For this review, take the finished solid that the model builds, in its own axes (mm). Round coordinates to 2 decimals unless told otherwise and drop trailing zeros. Order: outer loops, then holes, each group sorted by start corner. A loop starts at its lowest first (then second) coordinate and runs counter-clockwise, first axis right, second up.
```python
from build123d import *

# Parameters (mm, degrees)
SKETCH_1_R          = 1.5
EXTRUDE_1_DEPTH     = 1
SKETCH_3_R          = 1.5
CUT_EXTRUDE_1_DEPTH = 61.191781662
SKETCH_4_R          = 1.5
CUT_EXTRUDE_2_DEPTH = 61.191781662
CUT_EXTRUDE_3_DEPTH = 61.191781662


with BuildPart() as part:
    # Эскиз1 → Бобышка-Вытянуть1 (new body)
    with BuildSketch(Plane(origin=(0, 0, 0), x_dir=(1, 0, 0), z_dir=(0, 1, 0))):
        with BuildLine():
            Line((-48, -36.304966321), (48, -36.304966321))
            Line((48, -36.304966321), (48, 6.254720986))
            ThreePointArc((48, 6.254720986), (47.707106781, 6.961827767), (47, 7.254720986))
            Line((47, 7.254720986), (36.5, 7.254720986))
            ThreePointArc((36.5, 7.254720986), (29.428932188, 10.183653174), (26.5, 17.254720986))
            Line((26.5, 17.254720986), (26.5, 22.788381883))
            ThreePointArc((26.5, 22.788381883), (29.428932188, 29.859449695), (36.5, 32.788381883))
            Line((36.5, 32.788381883), (47, 32.788381883))
            ThreePointArc((47, 32.788381883), (47.707106781, 33.081275101), (48, 33.788381883))
            Line((48, 33.788381883), (48, 35.304966322))
            ThreePointArc((48, 35.304966322), (47.707106781, 36.012073103), (47, 36.304966322))
            Line((47, 36.304966322), (-47, 36.304966322))
            ThreePointArc((-47, 36.304966322), (-47.707106781, 36.012073103), (-48, 35.304966322))
            Line((-48, 35.304966322), (-48, 33.788381883))
            ThreePointArc((-48, 33.788381883), (-47.707106781, 33.081275101), (-47, 32.788381883))
            Line((-47, 32.788381883), (-36.5, 32.788381883))
            ThreePointArc((-36.5, 32.788381883), (-29.428932188, 29.859449695), (-26.5, 22.788381883))
            Line((-26.5, 22.788381883), (-26.5, 17.254720986))
            ThreePointArc((-26.5, 17.254720986), (-29.428932188, 10.183653174), (-36.5, 7.254720986))
            Line((-36.5, 7.254720986), (-47, 7.254720986))
            ThreePointArc((-47, 7.254720986), (-47.707106781, 6.961827767), (-48, 6.254720986))
            Line((-48, 6.254720986), (-48, -36.304966321))
        make_face()
        with Locations(Location((-21.397134942, 13.404966321, 0), (0, 0, 270))):
            Circle(SKETCH_1_R, mode=Mode.SUBTRACT)
        with Locations(Location((-21.397134942, 33.804966321, 0), (0, 0, 270))):
            Circle(SKETCH_1_R, mode=Mode.SUBTRACT)
        with Locations(Location((22.502865058, 13.404966321, 0), (0, 0, 270))):
            Circle(SKETCH_1_R, mode=Mode.SUBTRACT)
        with Locations(Location((22.502865058, 33.804966321, 0), (0, 0, 270))):
            Circle(SKETCH_1_R, mode=Mode.SUBTRACT)
        with BuildLine():
            Line((-19.5, -0.787211353), (-18, -1.787211353))
            Line((-18, -1.787211353), (18, -1.787211353))
            Line((18, -1.787211353), (19.5, -0.787211353))
            Line((19.5, -0.787211353), (19.5, 6.212788647))
            ThreePointArc((19.5, 6.212788647), (20.378679656, 8.334108991), (22.5, 9.212788647))
            Line((22.5, 9.212788647), (23.024503903, 9.212788647))
            ThreePointArc((23.024503903, 9.212788647), (24.348525199, 8.904807891), (25.400697774, 8.044100386))
            Line((25.400697774, 8.044100386), (32.206912135, -0.787211353))
            Line((32.206912135, -0.787211353), (37, -0.787211353))
            ThreePointArc((37, -0.787211353), (39.121320344, -1.665891009), (40, -3.787211353))
            Line((40, -3.787211353), (40, -8.287211353))
            Line((40, -8.287211353), (38, -10.787211353))
            Line((38, -10.787211353), (38, -20.787211353))
            Line((38, -20.787211353), (40, -23.287211353))
            Line((40, -23.287211353), (40, -27.787211353))
            ThreePointArc((40, -27.787211353), (39.121320344, -29.908531696), (37, -30.787211353))
            Line((37, -30.787211353), (19.5, -30.787211353))
            Line((19.5, -30.787211353), (18, -29.787211353))
            Line((18, -29.787211353), (-18, -29.787211353))
            Line((-18, -29.787211353), (-19.5, -30.787211353))
            Line((-19.5, -30.787211353), (-37, -30.787211353))
            ThreePointArc((-37, -30.787211353), (-39.121320344, -29.908531696), (-40, -27.787211353))
            Line((-40, -27.787211353), (-40, -23.287211353))
            Line((-40, -23.287211353), (-38, -20.787211353))
            Line((-38, -20.787211353), (-38, -10.787211353))
            Line((-38, -10.787211353), (-40, -8.287211353))
            Line((-40, -8.287211353), (-40, -3.787211353))
            ThreePointArc((-40, -3.787211353), (-39.121320344, -1.665891009), (-37, -0.787211353))
            Line((-37, -0.787211353), (-32.206912135, -0.787211353))
            Line((-32.206912135, -0.787211353), (-25.400697774, 8.044100386))
            ThreePointArc((-25.400697774, 8.044100386), (-24.348525199, 8.904807891), (-23.024503903, 9.212788647))
            Line((-23.024503903, 9.212788647), (-22.5, 9.212788647))
            ThreePointArc((-22.5, 9.212788647), (-20.378679656, 8.334108991), (-19.5, 6.212788647))
            Line((-19.5, 6.212788647), (-19.5, -0.787211353))
        make_face(mode=Mode.SUBTRACT)
    extrude(amount=EXTRUDE_1_DEPTH)

    # Эскиз3 → Вырез-Вытянуть1 (cut, through all)
    with BuildSketch(Plane.XZ):
        with Locations(Location((44, 33.82155076, 0), (0, 0, 270))):
            Circle(SKETCH_3_R)
        with Locations(Location((44, 0.766245183, 0), (0, 0, 270))):
            Circle(SKETCH_3_R)
        with Locations(Location((-44, 0.766245183, 0), (0, 0, 270))):
            Circle(SKETCH_3_R)
        with Locations(Location((-44, 33.82155076, 0), (0, 0, 270))):
            Circle(SKETCH_3_R)
    extrude(amount=-CUT_EXTRUDE_1_DEPTH, mode=Mode.SUBTRACT)

    # Эскиз4 → Вырез-Вытянуть2 (cut, through all)
    with BuildSketch(Plane.XZ):
        with Locations((-26.5, -8.260832856)):
            Circle(SKETCH_4_R)
        with Locations(Location((-8.5, -33.804966322, 0), (0, 0, 270))):
            Circle(SKETCH_4_R)
        with Locations(Location((8.5, -33.804966322, 0), (0, 0, 270))):
            Circle(SKETCH_4_R)
        with Locations((26.5, -8.260832856)):
            Circle(SKETCH_4_R)
    extrude(amount=-CUT_EXTRUDE_2_DEPTH, mode=Mode.SUBTRACT)

    # Эскиз6 → Вырез-Вытянуть3 (cut, through all)
    with BuildSketch(Plane(origin=(0, 1, 0), x_dir=(1, 0, 0), z_dir=(0, 1, 0))):
        with BuildLine():
            Line((-14.247312093, 18.245581007), (-8.247312093, 18.245581007))
            ThreePointArc((-8.247312093, 18.245581007), (-7.540205311, 17.952687789), (-7.247312093, 17.245581007))
            Line((-7.247312093, 17.245581007), (-7.247312093, 16.245581007))
            ThreePointArc((-7.247312093, 16.245581007), (-7.540205311, 15.538474226), (-8.247312093, 15.245581007))
            Line((-8.247312093, 15.245581007), (-14.247312093, 15.245581007))
            ThreePointArc((-14.247312093, 15.245581007), (-14.954418874, 15.538474226), (-15.247312093, 16.245581007))
            Line((-15.247312093, 16.245581007), (-15.247312093, 17.245581007))
            ThreePointArc((-15.247312093, 17.245581007), (-14.954418874, 17.952687789), (-14.247312093, 18.245581007))
        make_face()
    extrude(amount=-CUT_EXTRUDE_3_DEPTH, mode=Mode.SUBTRACT)


solid = part.part
```
Q1. Take a section at C-C, the plane x = -44. State the section outline as (y, z) points, plus the area to 3 significant figures.
Q2. Wall thickness on line 1 (Z direction, x = -36, y = 0.1); line 2 (X direction, y = 0.5, z = 4); line 3 (X direction, y = 0.35, z = -12.5): over which ranges is each line inside the solid? List them lowest first.
Q3. Take a section at A-A, the plane x = 8.5. State the section outline as (y, z) points.
Q4. Clearance check with a flat-ended pin moving along its axis: pin 1 (1.8 mm diameter, centred on x = 22.5, z = -33.8, fed in from +Y). State where the tip first meets the part, or that it passes through.
Q5. Take a section at B-B, the plane z = 26. State the section outline as (x, y) points, plus the area to 3 significant figures.
Q6. Take a section at D-D, the plane z = 15. State the section outline as (x, y) points.
Q7. Mouldability with a two-part tool opening along X and no side actions: class faces 1 (the face through (29.256, 0.493, -3.042)), 2 (the face through (-29.352, 0.493, -10.262)), 3 (the face through (29.507, 0.493, -10.106)), 4 (the face through (-27.695, 0.493, -9.167)) as +X half, -X half, draft (parallel to the pull), parting line (faces both ways), or undercut.
Working result:
1. outline: (0, -36.3) - (1, -36.3) - (1, -32.79) - (0, -32.79) - close; (0, -7.25) - (1, -7.25) - (1, -0.73) - (0, -0.73) - close; (0, 2.27) - (1, 2.27) - (1, 32.32) - (0, 32.32) - close; (0, 35.32) - (1, 35.32) - (1, 36.3) - (0, 36.3) - close
1. area: 41.1 mm2
2. line 1: z = -36.3 to -32.78, -7.27 to 0.79, 30.79 to 36.3
2. line 2: x = -48 to -40, 40 to 48
2. line 3: x = -27.7 to -22.59, -20.2 to 21.31, 23.7 to 27.7
3. outline: (0, -36.3) - (1, -36.3) - (1, -35.3) - (0, -35.3) - close; (0, -32.3) - (1, -32.3) - (1, 1.79) - (0, 1.79) - close; (0, 29.79) - (1, 29.79) - (1, 36.3) - (0, 36.3) - close
4. pin 1: passes through
5. outline: (-48, 0) - (-40, 0) - (-40, 1) - (-48, 1) - close; (40, 0) - (48, 0) - (48, 1) - (40, 1) - close
5. area: 16.0 mm2
6. outline: (-48, 0) - (-38, 0) - (-38, 1) - (-48, 1) - close; (38, 0) - (48, 0) - (48, 1) - (38, 1) - close
7. face 1: undercut
7. face 2: -X half
7. face 3: +X half
7. face 4: undercut
